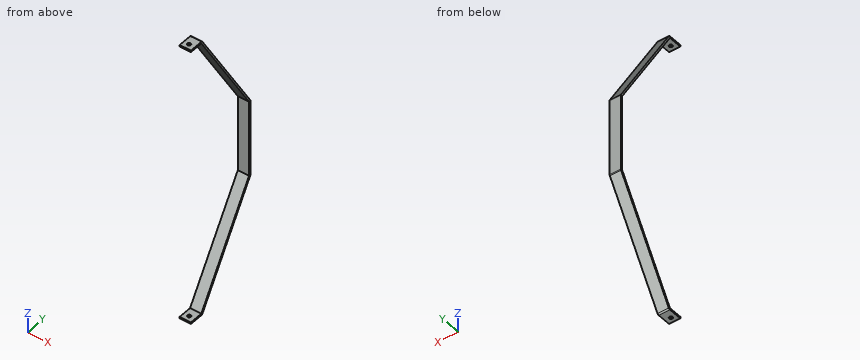
```python
from build123d import *

# Parameters (mm, degrees)
SM_BASE_FLANGE_1_DEPTH = 10
SKETCH_6_R             = 1.5
CUT_EXTRUDE_1_DEPTH    = 260.98076852


# Sheet-metal steps are written as plain solids
with BuildPart() as part:
    # Sketch 1 → 基体-法兰1 (new body)
    with BuildSketch(Plane(origin=(0, 0, 0), x_dir=(0, 0, -1), z_dir=(1, 0, 0))):
        with BuildLine():
            Line((124, -67), (124, -55.112166923))
            ThreePointArc((124, -55.112166923), (123.974439102, -55.014335437), (123.904290002, -54.941510557))
            Line((123.904290002, -54.941510557), (34.048016854, -0.029343633))
            ThreePointArc((34.048016854, -0.029343633), (33.997896617, -0.007475621), (33.943726853, 0))
            Line((33.943726853, 0), (-33.943726853, 0))
            ThreePointArc((-33.943726853, 0), (-33.997896617, -0.007475621), (-34.048016854, -0.029343633))
            Line((-34.048016854, -0.029343633), (-123.904290002, -54.941510557))
            ThreePointArc((-123.904290002, -54.941510557), (-123.974439102, -55.014335437), (-124, -55.112166923))
            Line((-124, -55.112166923), (-124, -67))
            Line((-124, -67), (-125.5, -67))
            Line((-125.5, -67), (-125.5, -55.112166923))
            ThreePointArc((-125.5, -55.112166923), (-125.282732364, -54.280599285), (-124.686465016, -53.661587806))
            Line((-124.686465016, -53.661587806), (-34.830191869, 1.250579117))
            ThreePointArc((-34.830191869, 1.250579117), (-34.404169846, 1.436457225), (-33.943726853, 1.5))
            Line((-33.943726853, 1.5), (33.943726853, 1.5))
            ThreePointArc((33.943726853, 1.5), (34.404169846, 1.436457225), (34.830191869, 1.250579117))
            Line((34.830191869, 1.250579117), (124.686465016, -53.661587806))
            ThreePointArc((124.686465016, -53.661587806), (125.282732364, -54.280599286), (125.5, -55.112166924))
            Line((125.5, -55.112166923), (125.5, -67))
            Line((125.5, -67), (124, -67))
        make_face()
    extrude(amount=SM_BASE_FLANGE_1_DEPTH)

    # 草图6 → 切除-拉伸1 (cut, through all)
    with BuildSketch(Plane.XY.offset(125.5)):
        with Locations((4.823171357, -62.280383367)):
            Circle(SKETCH_6_R)
    extrude(amount=-CUT_EXTRUDE_1_DEPTH, mode=Mode.SUBTRACT)


solid = part.part
```
Source: CAD feature listing. Evaluate the final solid. Frame: model axes, mm. Coordinates: 2 decimals unless noted, no trailing zeros. Write each loop counter-clockwise with the first axis right and the second up, starting at its lowest first coordinate (ties: lowest second). Pieces come first, ordered by that corner, then holes. Notation, with made-up numbers: M 39.25,-21.75 L 45.25,-21.75 A24 cw 45.25,14.25 Z; hole C 64.5,32.5 d6. An arc over 180 degrees is marked long. Answer as a JSON object with one key per item and string values.
1. Cut plane C-C on z = -7.5. Output: boundary loops of the cut face in (x, y), plus the area to 3 significant figures.
Evaluation:
{"outline": "M 0,0 L 10,0 L 10,1.5 L 0,1.5 Z", "area": "15.0 mm^2"}
2. Cut plane D-D on z = -40. Output: boundary loops of the cut face in (x, y).
Evaluation:
{"outline": "M 0,-3.67 L 10,-3.67 L 10,-1.91 L 0,-1.91 Z"}
3. Cut plane A-A on y = -36.5. Output: boundary loops of the cut face in (x, z), plus the area to 3 significant figures.
Evaluation:
{"outline": "M 0,-96.6 L 10,-96.6 L 10,-93.73 L 0,-93.73 Z; M 0,93.73 L 10,93.73 L 10,96.6 L 0,96.6 Z", "area": "57.5 mm^2"}
4. Cut plane B-B on x = 8. Output: boundary loops of the cut face in (y, z), plus the area to 3 significant figures.
Evaluation:
{"outline": "M -67,-125.5 L -55.11,-125.5 A1.7 ccw -53.66,-124.69 L 1.25,-34.83 A1.7 ccw 1.5,-33.94 L 1.5,33.94 A1.7 ccw 1.25,34.83 L -53.66,124.69 A1.7 ccw -55.11,125.5 L -67,125.5 L -67,124 L -55.11,124 A0.2 cw -54.94,123.9 L -0.03,34.05 A0.2 cw 0,33.94 L 0,-33.94 A0.2 cw -0.03,-34.05 L -54.94,-123.9 A0.2 cw -55.11,-124 L -67,-124 Z", "area": "458 mm^2"}
5. Contact query for flat-ended pins moving along their axis: P1, Ø2, axis at x = 6.5, y = -36, coming from the +Z side; P2, Ø5, axis at x = 5.5, z = 7.5, coming from the -Y side; P3, Ø6, axis at x = 3, y = -33.5, coming from the -Z side; P4, Ø2.5, axis at x = 4.82, y = -62.28, coming from the +Z side. Output: stop coordinate, or through.
Evaluation:
{"P1": "z = 97.42", "P2": "y = 0", "P3": "z = -96.6", "P4": "through"}
6. Ray query, L1, parallel to Z at x = 7.5, y = -63.5; L2, parallel to Y at x = 4.5, z = -28; L3, parallel to Z at x = 4.25, y = -15.5. Return the intervals inside material, ascending.
Evaluation:
{"L1": "-125.5 to -124, 124 to 125.5", "L2": "0 to 1.5", "L3": "-62.24 to -59.36, 59.36 to 62.24"}
